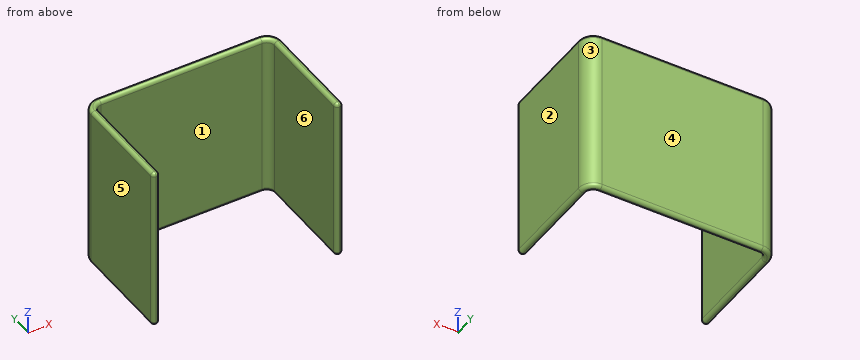
from build123d import *

# Parameters (mm, degrees)
SKETCH1_W           = 10.922
SKETCH1_H           = 0.4064
SKETCH1_W_2         = 0.4064
SKETCH1_H_2         = 6.223
BOSS_EXTRUDE1_DEPTH = 4.7625
FILLET1_R           = 0.8382
FILLET2_R           = 0.4318
FILLET3_R           = 0.2032


with BuildPart() as part:
    # Sketch1 → Boss-Extrude1 (new, symmetric)
    with BuildSketch(Plane.XY):
        Rectangle(SKETCH1_W, SKETCH1_H)
        with Locations((-5.2578, -3.3147)):
            Rectangle(SKETCH1_W_2, SKETCH1_H_2)
        with Locations((5.2578, -3.3147)):
            Rectangle(SKETCH1_W_2, SKETCH1_H_2)
    extrude(amount=BOSS_EXTRUDE1_DEPTH, both=True)

    # Fillet1
    fillet1_edges = [part.edges().sort_by_distance(p)[0] for p in [
        (-5.461, 0.2032, 0),
        (5.461, 0.2032, 0),
    ]]
    fillet(fillet1_edges, radius=FILLET1_R)

    # Fillet2
    fillet2_edges = [part.edges().sort_by_distance(p)[0] for p in [
        (5.0546, -0.2032, 0),
        (-5.0546, -0.2032, 0),
    ]]
    fillet(fillet2_edges, radius=FILLET2_R)

    # Fillet3
    fillet3_edges = [part.edges().sort_by_distance(p)[0] for p in [
        (-5.0546, -3.5306, -4.7625),
        (-5.2578, -6.4262, -4.7625),
        (5.461, -6.4262, 0),
        (5.0546, -6.4262, 0),
        (-5.0546, -6.4262, 0),
        (-5.461, -6.4262, 0),
        (-5.2578, -6.4262, 4.7625),
        (-5.0546, -3.5306, 4.7625),
        (-5.461, -3.5306, -4.7625),
        (-5.461, -3.5306, 4.7625),
        (5.461, -3.5306, -4.7625),
        (0, 0.2032, -4.7625),
        (5.215496904, -0.042303096, -4.7625),
        (-5.215496904, -0.042303096, -4.7625),
        (0, 0.2032, 4.7625),
        (5.461, -3.5306, 4.7625),
        (5.215496904, -0.042303096, 4.7625),
        (5.0546, -3.5306, 4.7625),
        (-5.215496904, -0.042303096, 4.7625),
        (5.2578, -6.4262, 4.7625),
        (0, -0.2032, -4.7625),
        (0, -0.2032, 4.7625),
        (-4.928128708, -0.329671292, -4.7625),
        (-4.928128708, -0.329671292, 4.7625),
        (4.928128708, -0.329671292, -4.7625),
        (4.928128708, -0.329671292, 4.7625),
        (5.2578, -6.4262, -4.7625),
        (5.0546, -3.5306, -4.7625),
    ]]
    fillet(fillet3_edges, radius=FILLET3_R - 0.0001)  # a hair under: the kernel refuses the full size


solid = part.part
Could you check a few things on this model? Use its own coordinates, in mm. Face numbers are marked on the shaded views. A direction names the side the tool comes from. Give positions to 0.01 mm unless a question says otherwise; leave off trailing zeros. Return JSON: item names as keys, results as strings. Group by question number.
Q1. Will this pin go through, and if not, where does the flat tip stop? pin 1 Ø2 at (x, z) = (3.5, 3.5) entering from -Y.
Q2. Please list where these lines run through material, in increasing order: line 1 along X through (y, z) = (-2, 3.25); line 2 along Y through (x, z) = (0.5, 4.5). Write a range as [from, to].
Q3. Which directions (+Z, -Z, +X, -X, +Y, -Y) give clear straight access to the entire face, cutting with the end or side of a thin tool? Please do the marked faces 1 and 2.
Q4. Thinking about a two-plate mould opening in X: for the marked faces 3, 4, 5 and 6, which applies, pulls with the +X half, pulls with the -X half, needs draft (parallel to the pull), parting line crosses it, or undercut?
Resolved:
{
 "1": {"pin 1": "stops at y = -0.2"},
 "2": {"line 1": "x = [-5.46, -5.05], [5.05, 5.46]", "line 2": "y = [-0.2, 0.2]"},
 "3": {"face 1": "+Z, -Z, -Y", "face 2": "+Z, -Z, +X, +Y, -Y"},
 "4": {"face 3": "pulls with the +X half", "face 4": "needs draft", "face 5": "pulls with the -X half", "face 6": "undercut"}
}
